Source: CAD feature listing. Evaluate the final solid. Frame: model axes, mm. A direction names the side the tool comes from. Give positions to 0.01 mm unless a question says otherwise; leave off trailing zeros. Write each loop counter-clockwise with the first axis right and the second up, starting at its lowest first coordinate (ties: lowest second). Pieces come first, ordered by that corner, then holes. Notation, with made-up numbers: M -12.5,-26.75 L 38.5,-26.75 A29 cw 38.5,3.25 Z; hole C 9,41 d8. An arc over 180 degrees is marked long. Return JSON: item names as keys, results as strings.
```python
from build123d import *

# Parameters (mm, degrees)
SKETCH1_W             = 20
SKETCH1_H             = 20
PCB_DEPTH             = 1
SKETCH3_W             = 20
SKETCH3_H             = 13
HEATSINK_DEPTH        = 3
SKETCH4_W             = 1.5
SKETCH4_H             = 1.5
HEATSINKPATTERN_DEPTH = 23.561028345
SKETCH5_W             = 20
SKETCH5_H             = 13.5
CAMERABASE_DEPTH      = 4.5
SKETCH6_R             = 6.5
CAMERACYLINDER_DEPTH  = 13.5
SKETCH7_R             = 8.75
LENS_DEPTH            = 4.3


with BuildPart() as part:
    # Sketch1 → PCB (new body)
    with BuildSketch(Plane(origin=(0, 0, 0), x_dir=(1, 0, 0), z_dir=(0, 1, 0))):
        Rectangle(SKETCH1_W, SKETCH1_H)
    extrude(amount=PCB_DEPTH)

    # Sketch3 → HeatSink (add)
    with BuildSketch(Plane.XZ):
        with Locations((0, -3.5)):
            Rectangle(SKETCH3_W, SKETCH3_H)
    extrude(amount=HEATSINK_DEPTH)

    # Sketch4 → HeatSinkPattern (cut, through all)
    with BuildSketch(Plane.ZY.offset(10)):
        with Locations((-1, -2.25)):
            Rectangle(SKETCH4_W, SKETCH4_H)
        with Locations((-3.5, -2.25)):
            Rectangle(SKETCH4_W, SKETCH4_H)
        with Locations((1.5, -2.25)):
            Rectangle(SKETCH4_W, SKETCH4_H)
        with Locations((-6, -2.25)):
            Rectangle(SKETCH4_W, SKETCH4_H)
        with Locations((-8.5, -2.25)):
            Rectangle(SKETCH4_W, SKETCH4_H)
    extrude(amount=-HEATSINKPATTERN_DEPTH, mode=Mode.SUBTRACT)

    # Sketch5 → CameraBase (add)
    with BuildSketch(Plane(origin=(0, 1, 0), x_dir=(1, 0, 0), z_dir=(0, 1, 0))):
        with Locations((0, 3.25)):
            Rectangle(SKETCH5_W, SKETCH5_H)
    extrude(amount=CAMERABASE_DEPTH)

    # Sketch6 → CameraCylinder (add)
    with BuildSketch(Plane(origin=(0, 5.5, 0), x_dir=(1, 0, 0), z_dir=(0, 1, 0))):
        with Locations(Location((0, 3.5, 0), (0, 0, 90))):
            Circle(SKETCH6_R)
    extrude(amount=CAMERACYLINDER_DEPTH)

    # Sketch7 → Lens (add)
    with BuildSketch(Plane(origin=(0, 19, 0), x_dir=(1, 0, 0), z_dir=(0, 1, 0))):
        with Locations(Location((0, 3.5, 0), (0, 0, 90))):
            Circle(SKETCH7_R)
    extrude(amount=LENS_DEPTH)


solid = part.part
```
1) Cut plane A-A, the plane z = -3.5. Return the cut outline in (x, y), then the cut area to 3 significant figures.
Numbers:
{"outline": "M -10,-1.5 L 10,-1.5 L 10,5.5 L 6.5,5.5 L 6.5,19 L 8.75,19 L 8.75,23.3 L -8.75,23.3 L -8.75,19 L -6.5,19 L -6.5,5.5 L -10,5.5 Z", "area": "391 mm²"}
2) Draft query along Z for faces 1 (the face through (0, -2, -0.25)), 2 (the face through (-10, 1, -2)), 3 (the face through (3.955, 12.156, 1.658)). Return one class per face: released by +Z, released by -Z, zero draft, split by the parting line, or undercut.
Numbers:
{"face 1": "undercut", "face 2": "zero draft", "face 3": "split by the parting line"}
3) Line query: line 1 (Z direction, x = 2, y = -1.75); line 2 (Y direction, x = 7.25, z = -0.5); line 3 (Y direction, x = -4.75, z = 6). Output: solid intervals per line, ascending. Write a range as [from, to].
Numbers:
{"line 1": "z = [-10, -9.25], [-7.75, -6.75], [-5.25, -4.25], [-2.75, -1.75], [-0.25, 0.75], [2.25, 3]", "line 2": "y = [-1.5, 5.5], [19, 23.3]", "line 3": "y = [0, 1]"}
4) Set-up query: faces 4 (the face through (0, -3, 0)), 5 (the face through (0, -2, 2.25)), 6 (the face through (0, 3, 3.5)), 7 (the face through (0, 0, 6)). Return all of +Z, -Z, +X, -X, +Y, -Y with unobstructed straight access to the full face (end or side cutting, diameter ignored); none if empty.
Numbers:
{"face 4": "+Z, -Z, +X, -X, -Y", "face 5": "+X, -X, -Y", "face 6": "+Z, +X, -X", "face 7": "+Z, +X, -X, -Y"}
5) Cut plane C-C, the plane y = 18.5. Return the cut outline in (x, z).
Numbers:
{"outline": "C 0,-3.5 d13"}
6) Contact query for flat-ended pins moving along their axis: pin 1 Ø1.5 at (x, y) = (-6, 9) entering from +Z; pin 2 Ø0.8 at (x, y) = (4, -2) entering from +Z; pin 3 Ø2 at (x, y) = (-4, 4) entering from +Z. Output: stop coordinate, or through.
Numbers:
{"pin 1": "stops at z = 0.33", "pin 2": "stops at z = 3", "pin 3": "stops at z = 3.5"}
